```python
from build123d import *

# Parameters (mm, degrees)
F0_R     = 36.25
F0_R_2   = 2.5
F1_DEPTH = 3
F3_DEPTH = 25
F4_R     = 5


with BuildPart() as f1:
    # F0 (on Front) → F1 (new body)
    with BuildSketch(Plane.XZ):
        Circle(F0_R)
        Circle(F0_R_2, mode=Mode.SUBTRACT)
    extrude(amount=F1_DEPTH)

    # F2 (on face) → F3 (cut)
    with BuildSketch(Plane.XZ.offset(3)):
        with BuildLine():
            ThreePointArc((-29.885841, -2.614672), (-21.213203, -21.213203), (-2.614672, -29.885841))
            Line((-2.614672, -29.885841), (-0.653668, -7.47146))
            ThreePointArc((-0.653668, -7.47146), (-5.303301, -5.303301), (-7.47146, -0.653668))
            Line((-7.47146, -0.653668), (-29.885841, -2.614672))
        make_face()
        with BuildLine():
            Line((-0.653668, 7.47146), (-2.614672, 29.885841))
            ThreePointArc((-2.614672, 29.885841), (-21.213203, 21.213203), (-29.885841, 2.614672))
            Line((-29.885841, 2.614672), (-7.47146, 0.653668))
            ThreePointArc((-7.47146, 0.653668), (-5.303301, 5.303301), (-0.653668, 7.47146))
        make_face()
        with BuildLine():
            Line((7.47146, 0.653668), (29.885841, 2.614672))
            ThreePointArc((29.885841, 2.614672), (21.213203, 21.213203), (2.614672, 29.885841))
            Line((2.614672, 29.885841), (0.653668, 7.47146))
            ThreePointArc((0.653668, 7.47146), (5.303301, 5.303301), (7.47146, 0.653668))
        make_face()
        with BuildLine():
            ThreePointArc((2.614672, -29.885841), (21.213203, -21.213203), (29.885841, -2.614672))
            Line((29.885841, -2.614672), (7.47146, -0.653668))
            ThreePointArc((7.47146, -0.653668), (5.303301, -5.303301), (0.653668, -7.47146))
            Line((0.653668, -7.47146), (2.614672, -29.885841))
        make_face()
    extrude(amount=-F3_DEPTH, mode=Mode.SUBTRACT)

    # F4
    f4_edges = [f1.edges().sort_by_distance(p)[0] for p in [
        (-0.653668, -1.5, 7.47146),
        (-7.47146, -1.5, 0.653668),
        (7.47146, -1.5, -0.653668),
        (0.653668, -1.5, -7.47146),
        (-7.47146, -1.5, -0.653668),
        (-0.653668, -1.5, -7.47146),
        (0.653668, -1.5, 7.47146),
        (7.47146, -1.5, 0.653668),
        (2.614672, -1.5, 29.885841),
        (-29.885841, -1.5, -2.614672),
        (29.885841, -1.5, -2.614672),
        (-2.614672, -1.5, -29.885841),
        (29.885841, -1.5, 2.614672),
        (-29.885841, -1.5, 2.614672),
        (2.614672, -1.5, -29.885841),
        (-2.614672, -1.5, 29.885841),
    ]]
    fillet(f4_edges, radius=F4_R)


solid = f1.part
```
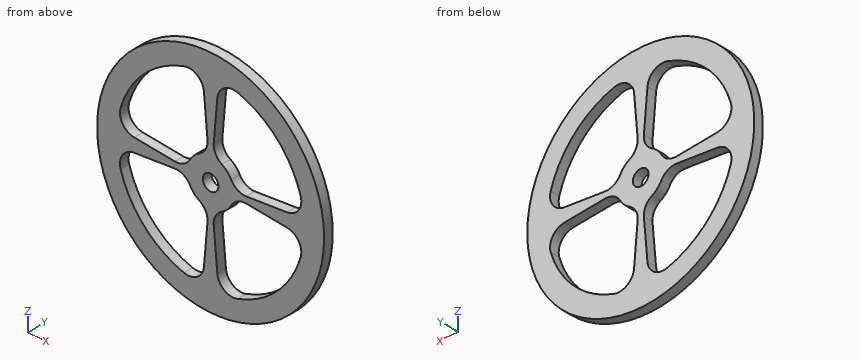
The listing builds one solid part. Answer for the finished solid, in the listing's coordinates (mm). Coordinates: 2 decimals unless noted, no trailing zeros. Order: outer loops, then holes, each group sorted by start corner. A loop starts at its lowest first (then second) coordinate and runs counter-clockwise, first axis right, second up. Notation, with made-up numbers: M -28,-33 L -9,-33 A23 ccw -9,3 Z; hole C 66.25,-14.75 d6. An arc over 180 degrees is marked long. Answer as a JSON object with one key per item and string values. Group by question number.
1. Section B-B on z = 0 is taken. Write down the section's boundary in (x, y), then the cut area to 4 significant figures.
2. Flat-ended cylindrical pins translate along their axes: P1, Ø1, axis at y = -1.5, z = -2, coming from the +X side; P2, Ø1, axis at x = 0, y = -2, coming from the -Z side; P3, Ø1, axis at x = 13, y = -2, coming from the -Z side; P4, Ø3, axis at x = 0, z = 0, coming from the +Y side. Find the tip coordinate at first contact, or state that the pin passes through.
3. Straight lines are drawn through the part: line 1 (X direction, y = -0.3, z = 21); line 2 (X direction, y = -1.75, z = 12); line 3 (Z direction, x = -7.5, y = -1.1). For each, find the intervals that lie inside material, in ascending order.
4. Section A-A on x = 0 is taken. Write down the section's boundary in (y, z), then the cut area to 4 significant figures.
5. Section D-D on z = 9.5 is taken. Write down the section's boundary in (x, y), then the cut area to 3 significant figures.
6. Section C-C on y = -2.15 is taken. State how many separate pieces and enclosed holes the cut face has, then the cut area to 3 significant figures.
Values follow:
{
 "1": {"outline": "M -36.25,-3 L -2.5,-3 L -2.5,0 L -36.25,0 Z; M 2.5,-3 L 36.25,-3 L 36.25,0 L 2.5,0 Z", "area": "202.5 mm2"},
 "2": {"P1": "x = 36.22", "P2": "z = -36.25", "P3": "z = -34.03", "P4": "through"},
 "3": {"line 1": "-29.55 to -21.42, -1.84 to 1.84, 21.42 to 29.55", "line 2": "-34.21 to -27.5, -1.05 to 1.05, 27.5 to 34.21", "line 3": "-35.47 to -28.95, -2.39 to 2.39, 28.95 to 35.47"},
 "4": {"outline": "M -3,-36.25 L 0,-36.25 L 0,-2.5 L -3,-2.5 Z; M -3,2.5 L 0,2.5 L 0,36.25 L -3,36.25 Z", "area": "202.5 mm2"},
 "5": {"outline": "M -34.98,-3 L -28.46,-3 L -28.46,0 L -34.98,0 Z; M -1.2,-3 L 1.2,-3 L 1.2,0 L -1.2,0 Z; M 28.46,-3 L 34.98,-3 L 34.98,0 L 28.46,0 Z", "area": "46.4 mm2"},
 "6": {"separate pieces": "1", "enclosed holes": "5", "area": "1,830 mm2"}
}
